from build123d import *

# Parameters (mm, degrees)
F1_DEPTH       = 20
F5_D           = 8
F5_DEPTH       = 30
F5_TIP         = 2.4034424761
F5_ON_F3_D     = 8
F5_ON_F3_DEPTH = 30
F5_ON_F3_TIP   = 2.4034424761
F5_ON_F4_D     = 8
F5_ON_F4_DEPTH = 30
F5_ON_F4_TIP   = 2.4034424761


with BuildPart() as f1:
    # F0 (on Right) → F1 (new body)
    with BuildSketch(Plane.YZ):
        Polygon((-376.1880215352, 0), (0, 0), (0, 80), (-330, 80), align=None)
    extrude(amount=F1_DEPTH)

    # F5
    with Locations(Plane(origin=(0, 0, 0), x_dir=(1, 0, 0), z_dir=(0, 0, -1))):
        with Locations((11, 325), (11, 130)):
            Hole(F5_D / 2, depth=F5_DEPTH)
            with Locations((0, 0, -(F5_DEPTH + F5_TIP / 2))):  # 118° drill point
                Cone(0, F5_D / 2, F5_TIP, mode=Mode.SUBTRACT)

    # F5 on F3
    with Locations(Plane(origin=(0, 0, 0), x_dir=(-1, 0, 0), z_dir=(0, 1, 0))):
        with Locations((-11, 15), (-11, 65)):
            Hole(F5_ON_F3_D / 2, depth=F5_ON_F3_DEPTH)
            with Locations((0, 0, -(F5_ON_F3_DEPTH + F5_ON_F3_TIP / 2))):  # 118° drill point
                Cone(0, F5_ON_F3_D / 2, F5_ON_F3_TIP, mode=Mode.SUBTRACT)

    # F5 on F4
    with Locations(Plane.XY.offset(80)):
        with Locations((11, -275), (11, -80)):
            Hole(F5_ON_F4_D / 2, depth=F5_ON_F4_DEPTH)
            with Locations((0, 0, -(F5_ON_F4_DEPTH + F5_ON_F4_TIP / 2))):  # 118° drill point
                Cone(0, F5_ON_F4_D / 2, F5_ON_F4_TIP, mode=Mode.SUBTRACT)


solid = f1.part
Check sheet for the modelled part. Datum: model origin and axes. Units: mm. A direction names the side the tool comes from. Give positions to 0.01 mm unless a question says otherwise; leave off trailing zeros. Write each loop counter-clockwise with the first axis right and the second up, starting at its lowest first coordinate (ties: lowest second). Pieces come first, ordered by that corner, then holes. Notation, with made-up numbers: M 85,65 L 96,65 A21 cw 96,100 Z; hole C 53.5,-11 d11. An arc over 180 degrees is marked long. Use one line per item in the form item = value.
(1) Tool access check on faces 4 (the cylindrical face through (9.154, -278.549, 64.79)), 5 (the cylindrical face through (10.479, -15.21, 18.966)), 6 (the cylindrical face through (11.521, -133.966, 15.21)). Record the directions out of +Z, -Z, +X, -X, +Y, -Y that give a thin tool (end or side, any length) a straight path to the whole face; none if there is none.
Answer block:
face_4 = +Z
face_5 = +Y
face_6 = -Z
(2) Depth check by flat-ended pin: P1, Ø12, axis at x = 15.5, z = 21, coming from the -Y side; P2, Ø6.5, axis at x = 11, z = 65, coming from the -Y side; P3, Ø2, axis at x = 17.5, z = 49, coming from the -Y side. Enter the tip coordinate at first touch or a pass-through.
Answer block:
P1 = -367.53
P2 = -340.54
P3 = -348.48
(3) Draft check along X on faces 1 (the flat face through (0, -191, 41)), 2 (the cylindrical face through (9.154, -321.451, 15.21)), 3 (the flat face through (10, -191, 0)). Enter one of: pulls with the +X half, pulls with the -X half, needs draft (parallel to the pull), parting line crosses it, or undercut.
Answer block:
face_1 = pulls with the -X half
face_2 = undercut
face_3 = needs draft
(4) Material ranges on line 1 along Z through (x, y) = (11, -7); line 2 along Z through (x, y) = (10, -17); line 3 along Y through (x, z) = (11, 23.5), recorded low to high.
Answer block:
line_1 = 0 to 11, 19 to 61, 69 to 80
line_2 = 0 to 11.13, 18.87 to 61.13, 68.87 to 80
line_3 = -362.62 to -329, -321 to -134, -126 to 0
(5) Section check A-A on z = 25. Record the boundary of the cut face in (x, y), plus the area to 3 significant figures.
Answer block:
outline = M 0,-361.75 L 20,-361.75 L 20,0 L 0,0 Z; hole C 11,-325 d8; hole C 11,-130 d8
area = 7,130 mm2
(6) Section check B-B on z = 41. Record the boundary of the cut face in (x, y).
Answer block:
outline = M 0,-352.52 L 20,-352.52 L 20,0 L 0,0 Z
